Can you work these out from the model? Positions are in its coordinate system, mm. Face numbers are marked on the shaded views. Round coordinates to 2 decimals unless told otherwise and drop trailing zeros. Loops run counter-clockwise (first coordinate to the right, second up) from the corner with the lowest first, then second, coordinate; pieces in that order, holes last.
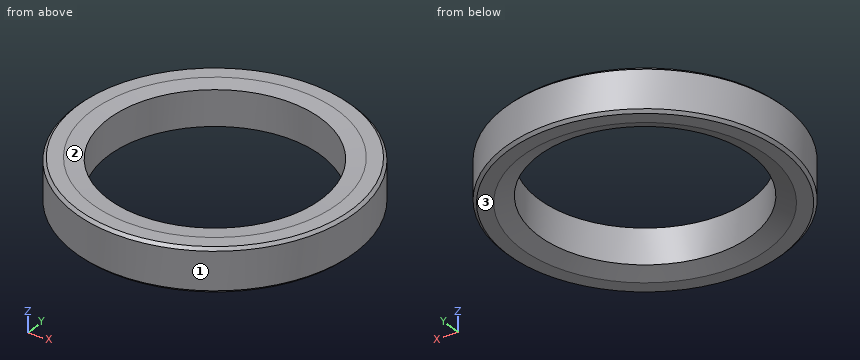
from build123d import *

# Parameters (mm, degrees)
CHAMFER1_SIZE = 0.5


with BuildPart() as part:
    # Sketch1 → Revolve1 (revolve)
    with BuildSketch(Plane(origin=(0, 0, 0), x_dir=(0, 0, -1), z_dir=(1, 0, 0)), mode=Mode.PRIVATE) as revolve1_sk:
        Polygon((-3.88315, 25), (3.88315, 25), (3.88315, 22), (2.682605307, 19), (-3.612740697, 19), (-3.88315, 22), align=None)
    revolve(revolve1_sk.sketch.rotate(Axis((0, 0, 4.95), (0, 0, -1)), 90), axis=Axis((0, 0, 4.95), (0, 0, -1)))

    # Chamfer1
    chamfer1_edges = [part.edges().sort_by_distance(p)[0] for p in [
        (-25, 0, 3.88315),
        (-25, 0, -3.88315),
    ]]
    chamfer(chamfer1_edges, length=CHAMFER1_SIZE)


solid = part.part
(1) If we mould it in two halves opening along X, with no side actions, what happens to the marked faces 1, 2 and 3? For each: released by +X, released by -X, zero draft, split by the parting line, or undercut.
Worked answers:
face 1: split by the parting line
face 2: undercut
face 3: zero draft
(2) Will these pins go through, and if not, where does the flat tip stop? P1, Ø12, axis at x = 4.5, y = 13.5, coming from the +Z side; P2, Ø23, axis at x = 0, y = 0, coming from the -Z side; P3, Ø10, axis at x = 15.5, y = -4, coming from the +Z side; P4, Ø3, axis at x = 18, z = -1.5, coming from the -Y side.
Worked answers:
P1: stops at z = 3.72
P2: passes through
P3: stops at z = 3.79
P4: stops at y = -18.78
(3) If we section it at A-A, the plane y = 0: List the corners of the cut face in (x, z) for me, then the cut area to 3 significant figures.
Worked answers:
outline: (-25, -3.38) - (-24.5, -3.88) - (-22, -3.88) - (-19, -2.68) - (-19, 3.61) - (-22, 3.88) - (-24.5, 3.88) - (-25, 3.38) - close; (19, -2.68) - (22, -3.88) - (24.5, -3.88) - (25, -3.38) - (25, 3.38) - (24.5, 3.88) - (22, 3.88) - (19, 3.61) - close
area: 88.3 mm2
(4) If I drill on line 1 (Y direction, x = 0, z = -0.75); line 2 (Y direction, x = -8, z = -2.5); line 3 (X direction, y = 14, z = 2), over which ranges is the centre line in solid material (lowest first)?
Worked answers:
line 1: y = -25 to -19, 19 to 25
line 2: y = -23.69 to -17.23, 17.23 to 23.69
line 3: x = -20.71 to -12.85, 12.85 to 20.71
(5) If we section it at C-C, the plane z = 2.75: List the corners of the cut face in (x, y) for me, then the cut area to 3 significant figures.
Worked answers:
outline: circle Ø50 at (0, 0); hole circle Ø38 at (0, 0)
area: 829 mm2
